from build123d import *

# Parameters (mm, degrees)
SKETCH1_R           = 5.6
BOSS_EXTRUDE1_DEPTH = 7.2
SKETCH2_R           = 1.5
CUT_EXTRUDE1_DEPTH  = 24.787391618


with BuildPart() as part:
    # Sketch1 → Boss-Extrude1 (new body)
    with BuildSketch(Plane.XY):
        with BuildLine():
            Line((10, 0), (17, 0))
            Line((17, 0), (17, -5))
            Line((17, -5), (-17, -5))
            Line((-17, -5), (-17, 0))
            Line((-17, 0), (-10, 0))
            Line((-10, 0), (-10, 5))
            ThreePointArc((-10, 5), (0, 15), (10, 5))
            Line((10, 5), (10, 0))
        make_face()
        with Locations((0, 5)):
            Circle(SKETCH1_R, mode=Mode.SUBTRACT)
    extrude(amount=BOSS_EXTRUDE1_DEPTH)

    # Sketch2 → Cut-Extrude1 (cut, through all)
    with BuildSketch(Plane(origin=(0, 0, 0), x_dir=(1, 0, 0), z_dir=(0, 1, 0))):
        with Locations(Location((13.5, -3.6, 0), (0, 0, 180))):
            Circle(SKETCH2_R)
        with Locations((-13.5, -3.6)):
            Circle(SKETCH2_R)
    extrude(amount=-CUT_EXTRUDE1_DEPTH, mode=Mode.SUBTRACT)


solid = part.part
The model under review builds one solid part; all positions refer to its coordinate system, in mm. A direction names the side the tool comes from. Round coordinates to 2 decimals unless told otherwise and drop trailing zeros. Write each loop counter-clockwise with the first axis right and the second up, starting at its lowest first coordinate (ties: lowest second). Pieces come first, ordered by that corner, then holes. Notation, with made-up numbers: (78, -33.5) - (89, -33.5) arc R24 cw to (89, 0.5) - close; hole circle Ø3 at (-12, 33.5). An arc over 180 degrees is marked (long way). One line per item, written item: value. Start each with the question number.
1. Consider section C-C on y = 3.75. Write out the cut boundary in (x, z), and give its area (3 significant figures).
2. Consider section D-D on z = 6. Write out the cut boundary in (x, y).
3. Clearance check with flat-ended pins moving along their axes: P1, Ø3.5, axis at x = 12.5, z = 4.5, coming from the +Y side; P2, Ø6, axis at x = 10, y = 7.5, coming from the -Z side; P3, Ø4, axis at y = 2.5, z = 4, coming from the +X side; P4, Ø3, axis at y = 7.5, z = 3.5, coming from the +X side. State where each tip first meets the part, or that it passes through.
4. Consider section B-B on x = -13.5. Write out the cut boundary in (y, z), and give its area (3 significant figures).
5. To check wall thickness, follow L1, parallel to X at y = -2.25, z = 3.5; L2, parallel to Y at x = 0, z = 5.5; L3, parallel to Z at x = -13.5, y = -2.65. State the ranges of each line that lie inside material, in increasing order. Write a range as from..to.
6. The part is to be moulded in two halves that separate along X. For faces 1 (the face through (10, 3, 4)), 2 (the face through (-10, 2, 4)), 3 (the face through (-14.7, -2.5, 4.5)), say which applies: released by +X, released by -X, zero draft, split by the parting line, or undercut.
7. Machinability: for faces 4 (the face through (-14, 0, 2)), 5 (the face through (13, 0, 2)), 6 (the face through (17, -2, 4)), which of the approach directions +Z, -Z, +X, -X, +Y, -Y give a long, thin tool a straight path to every point of the face, cutting with its end or side? Answer none if there is none.
8. Consider section A-A on z = 3.6. Write out the cut boundary in (x, y), and give its area (3 significant figures).
Checks:
1. outline: (-10, 0) - (-5.46, 0) - (-5.46, 7.2) - (-10, 7.2) - close; (5.46, 0) - (10, 0) - (10, 7.2) - (5.46, 7.2) - close
1. area: 65.4 mm^2
2. outline: (-17, -5) - (17, -5) - (17, 0) - (10, 0) - (10, 5) arc R10 ccw to (-10, 5) - (-10, 0) - (-17, 0) - close; hole circle Ø11.2 at (0, 5)
3. P1: stops at y = 0
3. P2: stops at z = 0
3. P3: stops at x = 10
3. P4: stops at x = 9.95
4. outline: (-5, 0) - (0, 0) - (0, 2.1) - (-5, 2.1) - close; (-5, 5.1) - (0, 5.1) - (0, 7.2) - (-5, 7.2) - close
4. area: 21.0 mm^2
5. L1: x = -17..-15, -12..12, 15..17
5. L2: y = -5..-0.6, 10.6..15
5. L3: z = 0..2.1, 5.1..7.2
6. face 1: released by +X
6. face 2: released by -X
6. face 3: undercut
7. face 4: +Z, -Z, -X, +Y
7. face 5: +Z, -Z, +X, +Y
7. face 6: +Z, -Z, +X, +Y, -Y
8. outline: (-17, -5) - (-15, -5) - (-15, 0) - (-17, 0) - close; (-12, -5) - (12, -5) - (12, 0) - (10, 0) - (10, 5) arc R10 ccw to (-10, 5) - (-10, 0) - (-12, 0) - close; (15, -5) - (17, -5) - (17, 0) - (15, 0) - close; hole circle Ø11.2 at (0, 5)
8. area: 299 mm^2
